Verification items for the finished model (mm, model axes). A direction names the side the tool comes from. Coordinates: 2 decimals unless noted, no trailing zeros. Order: outer loops, then holes, each group sorted by start corner. A loop starts at its lowest first (then second) coordinate and runs counter-clockwise, first axis right, second up. Notation, with made-up numbers: (-10, 2.25) -> (35, 2.25) arc R13 cw to (35, 14.25) -> close; hole circle Ø5 at (23.5, 26). An arc over 180 degrees is marked (long way). Write each question's results on one line, items separated by ' | '. Start each with the question number.
(1) Cross-section at A-A on y = -85. Enter the section's corners in (x, z) (1 decimal), and give its area (3 significant figures).
(2) Go/stop test with flat-tipped pins: pin 1 (8 mm diameter, centred on x = 0, z = 265.25, fed in from -Y); pin 2 (12 mm diameter, centred on x = -41, y = -313.5, fed in from -Z); pin 3 (3 mm diameter, centred on y = -179.5, z = 95.5, fed in from +X). Record where each tip stops, or that it passes through.
(3) Thickness scan on probe 1 along Y at (x, z) = (188, -102); probe 2 along X at (y, z) = (-345, -145); probe 3 along X at (y, z) = (-601.5, 216). Record the ranges inside material, lowest first. Write a range as [from, to].
(4) Draft check along Z on faces 1 (the flat face through (-3, -679.45, 3)), 2 (the cylindrical face through (272.786, 12.522, -12.005)), 3 (the flat face through (167, 22.225, 186)). Enter one of: +Z half, -Z half, draft (parallel to the pull), parting line (faces both ways), or undercut.
(5) Set-up check for faces 4 (the cylindrical face through (-53.34, -331.84, 240.21)), 5 (the flat face through (-241, 25.4, -80)), 6 (the cylindrical face through (-54.72, 23.83, 246.41)): record each of +Z, -Z, +X, -X, +Y, -Y from which the full face is reachable in a straight line by a thin tool's end or side.
Autodesk Inventor part; units mm, degrees
ref_plane "YZ Plane" through (0, 0, 0) normal (1, 0, 0) x (0, 1, 0)
ref_plane "XZ Plane" through (0, 0, 0) normal (0, 1, 0) x (-1, 0, 0)
ref_plane "XY Plane" through (0, 0, 0) normal (0, 0, 1) x (1, 0, 0)
sketch "Sketch1" plane through (0, 0, 0) normal (0, 1, 0) x (-1, 0, 0)
  circle A0 centre (0, 0) radius 273.05
  circle A1 centre (0, 0) radius 242.8875
  dimension "d0" = 546.1
  dimension "d1" = 485.775
extrude "Extrusion1" add sketch "Sketch1" along normal blind 25.4
sketch "Sketch2" plane through (0, 25.4, 0) normal (0, 1, 0) x (1, 0, 0)
  circle A0 centre (0, 0) radius 247.65
  circle A1 centre (0, 0) radius 252.4125
  dimension "d4" = 495.3
  dimension "d5" = 504.825
extrude "Extrusion2" cut sketch "Sketch2" against normal blind 3.175
sketch "Sketch3" plane through (0, 25.4, 0) normal (0, 1, 0) x (1, 0, 0)
  line L0 (0, 0) -> (-265.25, 0) construction
  dimension "d8" = 265.25
hole "Hole1" at (-265.25, 25.4, 0) direction (0, -1, 0) diameter 6.9088 end up to surface
pattern_circular "Circular Pattern1" count 12 over 360 about axis through (0, -10, 0) along (0, 1, 0) of "Hole1"
sketch "Sketch4" plane through (0, 0, 0) normal (0, -1, 0) x (1, 0, 0)
  circle A0 centre (0, 0) radius 242.8875
  circle A1 centre (0, 0) radius 246.0625
  dimension "d19" = 485.775
  dimension "d20" = 492.125
extrude "Extrusion3" add sketch "Sketch4" along normal blind 679.45
sketch "Sketch8" plane through (0, -679.45, 0) normal (0, -1, 0) x (1, 0, 0)
  circle A0 centre (0, 0) radius 246.0625
  dimension "d45" = 492.125
extrude "Extrusion6" add sketch "Sketch8" against normal blind 6.35
fillet "Fillet1" radius 6.35 2 edges at (-246.0625, -679.45, 0) (-242.8875, -673.1, 0)
properties part number "vacuum jacket long" material "Aluminum 6061"
Results are:
1) outline: circle Ø492.1 at (0, 0); hole circle Ø485.8 at (0, 0) | area: 4,880 mm2
2) pin 1: stops at y = 0 | pin 2: stops at z = -243.56 | pin 3: stops at x = 227.4
3) probe 1: y = [-679.45, -673.1] | probe 2: x = [-198.8, -194.86], [194.86, 198.8] | probe 3: x = [-117.86, -111.08], [111.08, 117.86]
4) face 1: draft | face 2: parting line | face 3: undercut
5) face 4: -Y | face 5: +Z, -Z, +X, -X, +Y | face 6: +Y
